from build123d import *

# Parameters (mm, degrees)
SKETCH1_R           = 3
BOSS_EXTRUDE1_DEPTH = 5
SKETCH2_W           = 70
SKETCH2_H           = 5
BOSS_EXTRUDE2_DEPTH = 70
CUT_EXTRUDE1_DEPTH  = 20
SKETCH4_R           = 15.5
CUT_EXTRUDE2_DEPTH  = 10
CUT_EXTRUDE6_REACH  = 77
SKETCH8_W           = 20
SKETCH8_H           = 20
SKETCH9_W           = 40
SKETCH9_H           = 5
CUT_EXTRUDE7_DEPTH  = 30
SKETCH10_R          = 2.5
CUT_EXTRUDE8_DEPTH  = 5


with BuildPart() as part:
    # Sketch1 → Boss-Extrude1 (new body)
    with BuildSketch(Plane(origin=(0, 0, 0), x_dir=(1, 0, 0), z_dir=(0, 1, 0))):
        Polygon((-35, -40), (-20, -40), (-20, -70), (20, -70), (20, -40), (35, -40), (60, -40), (60, 39), (-60, 39), (-60, -40), align=None)
        with Locations((49.796460718, 28.75)):
            Circle(SKETCH1_R, mode=Mode.SUBTRACT)
        with Locations((49.796460718, -28.75)):
            Circle(SKETCH1_R, mode=Mode.SUBTRACT)
        with Locations((0, -57.5)):
            Circle(SKETCH1_R, mode=Mode.SUBTRACT)
        with Locations((-49.796460718, -28.75)):
            Circle(SKETCH1_R, mode=Mode.SUBTRACT)
        with Locations((-49.796460718, 28.75)):
            Circle(SKETCH1_R, mode=Mode.SUBTRACT)
    extrude(amount=BOSS_EXTRUDE1_DEPTH)

    # Sketch2 → Boss-Extrude2 (add)
    with BuildSketch(Plane(origin=(0, 5, 0), x_dir=(1, 0, 0), z_dir=(0, 1, 0))):
        with Locations((0, 16.5)):
            Rectangle(SKETCH2_W, SKETCH2_H)
    extrude(amount=BOSS_EXTRUDE2_DEPTH)

    # Sketch3 → Cut-Extrude1 (cut)
    with BuildSketch(Plane(origin=(0, 0, -19), x_dir=(-1, 0, 0), z_dir=(0, 0, -1))):
        with BuildLine():
            ThreePointArc((-35, 40.000002437), (-24.74873648, 64.748738203), (0, 75))
            Line((0, 75), (-35, 75))
            Line((-35, 75), (-35, 40.000002437))
        make_face()
        with BuildLine():
            Line((35, 40.000002339), (35, 75))
            Line((35, 75), (0, 75))
            ThreePointArc((0, 75), (24.748736514, 64.748738169), (35, 40.000002339))
        make_face()
    extrude(amount=-CUT_EXTRUDE1_DEPTH, mode=Mode.SUBTRACT)

    # Sketch4 → Cut-Extrude2 (cut)
    with BuildSketch(Plane.XY.offset(-14)):
        with Locations((0, 40)):
            Circle(SKETCH4_R)
    extrude(amount=-CUT_EXTRUDE2_DEPTH, mode=Mode.SUBTRACT)

    # Sketch8 → Cut-Extrude6 (cut, up to next)
    with BuildSketch(Plane.XZ, mode=Mode.PRIVATE) as cut_extrude6_sk1:
        Rectangle(SKETCH8_W, SKETCH8_H)
    cut_extrude6_tool1 = extrude(cut_extrude6_sk1.sketch, amount=-CUT_EXTRUDE6_REACH, mode=Mode.PRIVATE) & part.part
    add(cut_extrude6_tool1.solids().sort_by_distance((0, 0, 0))[0], mode=Mode.SUBTRACT)

    # Sketch9 → Cut-Extrude7 (cut)
    with BuildSketch(Plane.XY.offset(70)):
        with Locations((0, 2.5)):
            Rectangle(SKETCH9_W, SKETCH9_H)
    extrude(amount=-CUT_EXTRUDE7_DEPTH, mode=Mode.SUBTRACT)

    # Sketch10 → Cut-Extrude8 (cut)
    with BuildSketch(Plane(origin=(0, 0, -19), x_dir=(-1, 0, 0), z_dir=(0, 0, -1))):
        with Locations((14.142135624, 54.142135624)):
            Circle(SKETCH10_R)
        with Locations((14.142135624, 25.857864376)):
            Circle(SKETCH10_R)
        with Locations((-14.142135624, 25.857864376)):
            Circle(SKETCH10_R)
        with Locations((-14.142135624, 54.142135624)):
            Circle(SKETCH10_R)
    extrude(amount=-CUT_EXTRUDE8_DEPTH, mode=Mode.SUBTRACT)


solid = part.part
Design review of the part built by this model. Coordinates are the model's own, in mm. A direction names the side the tool comes from. Give positions to 0.01 mm unless a question says otherwise; leave off trailing zeros. Order: outer loops, then holes, each group sorted by start corner. A loop starts at its lowest first (then second) coordinate and runs counter-clockwise, first axis right, second up.
1. Add section C-C, the plane x = 49.5. State the section outline as (y, z) points, then the cut area to 3 significant figures.
Solution:
outline: (0, -39) - (5, -39) - (5, -31.74) - (0, -31.74) - close; (0, -25.76) - (5, -25.76) - (5, 25.76) - (0, 25.76) - close; (0, 31.74) - (5, 31.74) - (5, 40) - (0, 40) - close
area: 335 mm2
2. Mouldability with a two-part tool opening along Z and no side actions: class faces 1 (the flat face through (-1, 2, 40)), 2 (the cylindrical face through (-52.794, 2.465, 28.618)), 3 (the flat face through (0, 2, 10)), 4 (the flat face through (-60, 2, 0)) as +Z half, -Z half, draft (parallel to the pull), parting line (faces both ways), or undercut.
Solution:
face 1: +Z half
face 2: undercut
face 3: undercut
face 4: draft
3. Tool access review of faces 5 (the flat face through (-10, 2, 0)), 6 (the flat face through (0, 24, -14)), 7 (the flat face through (35, 22, -16)), 8 (the flat face through (60, 2, 1)), 9 (the flat face through (-35, 22, -16)): name each direction out of +Z, -Z, +X, -X, +Y, -Y from which nothing blocks a thin tool from reaching the whole face with its end or side.
Solution:
face 5: +Y, -Y
face 6: +Z, +X, -X, +Y
face 7: +Z, -Z, +X, +Y
face 8: +Z, -Z, +X, +Y, -Y
face 9: +Z, -Z, -X, +Y
4. To check wall thickness, follow L1, parallel to X at y = 2.55, z = 28.75; L2, parallel to Y at x = -11.5, z = -34.5; L3, parallel to Z at x = -32, y = 20.5. State the ranges of each line that lie inside material, in increasing order.
Solution:
L1: x = -60 to -52.8, -46.8 to 46.8, 52.8 to 60
L2: y = 0 to 5
L3: z = -19 to -14
5. Add section A-A, the plane z = 28.75. State the section outline as (x, y) points.
Solution:
outline: (-60, 0) - (-52.8, 0) - (-52.8, 5) - (-60, 5) - close; (-46.8, 0) - (46.8, 0) - (46.8, 5) - (-46.8, 5) - close; (52.8, 0) - (60, 0) - (60, 5) - (52.8, 5) - close
6. For pin 1 Ø5 at (x, z) = (-49.8, 28.75) entering from +Y; pin 2 Ø2.5 at (y, z) = (16.5, -16.5) entering from +X; pin 3 Ø8 at (x, y) = (14.14, 54.14) entering from -Z; pin 4 Ø4 at (y, z) = (59, -15) entering from +X, all flat-tipped, find the tip position at first contact; note any pin that passes through.
Solution:
pin 1: passes through
pin 2: stops at x = 35
pin 3: stops at z = -19
pin 4: stops at x = 30.59
7. Add section B-B, the plane z = 4.5. State the section outline as (x, y) points, then the cut area to 3 significant figures.
Solution:
outline: (-60, 0) - (-10, 0) - (-10, 5) - (-60, 5) - close; (10, 0) - (60, 0) - (60, 5) - (10, 5) - close
area: 500 mm2
8. Add section D-D, the plane y = 20. State the section outline as (x, z) points, then the cut area to 3 significant figures.
Solution:
outline: (-35, -19) - (35, -19) - (35, -14) - (-35, -14) - close
area: 350 mm2
